from build123d import *

# Parameters (mm, degrees)
ESQUISSE1_R             = 7
ESQUISSE1_R_2           = 1.8
BOSS_EXTRU_1_DEPTH      = 8
ESQUISSE2_R             = 13.4
ENL_V_MAT_EXTRU_1_DEPTH = 9
ESQUISSE3_R             = 2
ENL_V_MAT_EXTRU_2_DEPTH = 12
CHANFREIN1_SIZE         = 1


with BuildPart() as part:
    # Esquisse1 → Boss.-Extru.1 (new body)
    with BuildSketch(Plane.XY):
        with BuildLine():
            Line((-20, 0), (-20, -25))
            Line((-20, -25), (20, -25))
            Line((20, -25), (20, 0))
            ThreePointArc((20, 0), (0, 20), (-20, 0))
        make_face()
        Circle(ESQUISSE1_R, mode=Mode.SUBTRACT)
        with Locations((0, 10)):
            Circle(ESQUISSE1_R_2, mode=Mode.SUBTRACT)
        with Locations((10, 0)):
            Circle(ESQUISSE1_R_2, mode=Mode.SUBTRACT)
        with Locations((0, -10)):
            Circle(ESQUISSE1_R_2, mode=Mode.SUBTRACT)
        with Locations((-10, 0)):
            Circle(ESQUISSE1_R_2, mode=Mode.SUBTRACT)
    extrude(amount=BOSS_EXTRU_1_DEPTH)

    # Esquisse2 → Enlèv. mat.-Extru.1 (cut, through all)
    with BuildSketch(Plane.XY.offset(8)):
        Circle(ESQUISSE2_R)
    extrude(amount=-ENL_V_MAT_EXTRU_1_DEPTH, mode=Mode.SUBTRACT)

    # Esquisse3 → Enlèv. mat.-Extru.2 (cut)
    with BuildSketch(Plane.XZ.offset(25)):
        with Locations((-15, 4)):
            Circle(ESQUISSE3_R)
        with Locations((15, 4)):
            Circle(ESQUISSE3_R)
    extrude(amount=-ENL_V_MAT_EXTRU_2_DEPTH, mode=Mode.SUBTRACT)

    # Chanfrein1
    chanfrein1_edges = [part.edges().sort_by_distance(p)[0] for p in [
        (-17, -25, 4),
        (13, -25, 4),
    ]]
    chamfer(chanfrein1_edges, length=CHANFREIN1_SIZE)


solid = part.part
The model under review builds one solid part; all positions refer to its coordinate system, in mm. A direction names the side the tool comes from. Round coordinates to 2 decimals unless told otherwise and drop trailing zeros. Write each loop counter-clockwise with the first axis right and the second up, starting at its lowest first coordinate (ties: lowest second). Pieces come first, ordered by that corner, then holes. Notation, with made-up numbers: M -39.5,4 L -23.5,4 A18 ccw -23.5,34 Z; hole C 82.25,48 d2. An arc over 180 degrees is marked long. Use a Markdown table: item, result. Add a question column.
Q1. The part is to be moulded in two halves that separate along Z. For faces 1 (the face through (-15, -19, 2)), 2 (the face through (-9, -12, 0)), 3 (the face through (20, -13, 4)), say which applies: pulls with the +Z half, pulls with the -Z half, needs draft (parallel to the pull), parting line crosses it, or undercut.
Q2. To check wall thickness, follow line 1 (Z direction, x = 15, y = -20.25); line 2 (Y direction, x = 4, z = 7); line 3 (X direction, y = -12, z = 6). State the ranges of each line that lie inside material, in increasing order.
Q3. We need section B-B, the plane y = -2.5. State the section outline as (x, z) points, plus the area to 3 significant figures.
Q4. Insertion check: pin 1 (2 mm diameter, centred on x = 15, z = 4.5, fed in from -Y); pin 2 (3.5 mm diameter, centred on x = 15, z = 4, fed in from +Y). Each pin has a flat end and moves straight along its axis. Give the tip position at first contact, or say it passes through.
Q5. We need section C-C, the plane x = -15. State the section outline as (y, z) points, plus the area to 3 significant figures.
Q6. Machinability: for faces 4 (the face through (-20, -12, 4)), 5 (the face through (13.4, -18.6, 2.8)), which of the approach directions +Z, -Z, +X, -X, +Y, -Y give a long, thin tool a straight path to every point of the face, cutting with its end or side? Answer none if there is none.
Q7. We need section A-A, the plane x = 0. State the section outline as (y, z) points.
Findings below:
| question | item | result |
|---|---|---|
| 1 | face 1 | undercut |
| 1 | face 2 | pulls with the -Z half |
| 1 | face 3 | needs draft |
| 2 | line 1 | z = 0 to 2, 6 to 8 |
| 2 | line 2 | y = -25 to -12.79, 12.79 to 19.6 |
| 2 | line 3 | x = -20 to -5.96, 5.96 to 20 |
| 3 | outline | M -20,0 L -13.16,0 L -13.16,8 L -20,8 Z; M 13.16,0 L 20,0 L 20,8 L 13.16,8 Z |
| 3 | area | 109 mm² |
| 4 | pin 1 | stops at y = -13 |
| 4 | pin 2 | stops at y = 14.98 |
| 5 | outline | M -25,0 L 13.23,0 L 13.23,8 L -25,8 L -25,7 L -24,6 L -13,6 L -13,2 L -24,2 L -25,1 Z |
| 5 | area | 257 mm² |
| 6 | face 4 | +Z, -Z, -X, +Y, -Y |
| 6 | face 5 | -Y |
| 7 | outline | M -25,0 L -13.4,0 L -13.4,8 L -25,8 Z; M 13.4,0 L 20,0 L 20,8 L 13.4,8 Z |
